```python
from build123d import *

# Parameters (mm, degrees)
SKETCH_4_R             = 12.471621376
EXTRUDE_2_DEPTH        = 8
SKETCH_6_R             = 8.974783973
EXTRUDE_3_DEPTH        = 8
HOLE_WIZARD_M201_D     = 20.25
HOLE_WIZARD_M201_DEPTH = 10
HOLE_WIZARD_M201_TIP   = 6.083713768


with BuildPart() as part:
    # Эскиз2 → Повернуть1 (revolve)
    with BuildSketch(Plane.XY):
        with BuildLine():
            Line((-4.5, 0.130191103), (-7.868865891, 0.130191103))
            ThreePointArc((-7.868865891, 0.130191103), (-9.846990335, 0.874747979), (-10.843230675, 2.73884198))
            Line((-10.843230675, 2.73884198), (-12.471621376, 15.115075065))
            Line((-12.471621376, 15.115075065), (-12.471621376, 23.115075065))
            Line((-12.471621376, 23.115075065), (-14.984883962, 23.115075065))
            Line((-14.984883962, 23.115075065), (-14.984883962, 29.115075065))
            Line((-14.984883962, 29.115075065), (-13.983803036, 29.115075065))
            Line((-13.983803036, 29.115075065), (-13.983803036, 32.115075065))
            Line((-13.983803036, 32.115075065), (-11.48027645, 32.115075065))
            Line((-11.48027645, 32.115075065), (-11.48027645, 37.115075065))
            Line((-11.48027645, 37.115075065), (-8.974783973, 37.115075065))
            Line((-8.974783973, 37.115075065), (-8.974783973, 23.115075065))
            Line((-8.974783973, 23.115075065), (-6.974783973, 23.115075065))
            Line((-6.974783973, 23.115075065), (-6.974783973, 18.115075065))
            Line((-6.974783973, 18.115075065), (-4.449353589, 18.115075065))
            Line((-4.449353589, 18.115075065), (-4.490567157, 3.479857527))
            Line((-4.490567157, 3.479857527), (-6.488062408, 3.489211927))
            Line((-6.488062408, 3.489211927), (-6.49087648, 2.489915788))
            Line((-6.49087648, 2.489915788), (-4.493381229, 2.480561388))
            Line((-4.493381229, 2.480561388), (-4.5, 0.130191103))
        make_face()
    revolve(axis=Axis((0, 0, 0), (0, 1, 0)))

    # Эскиз4 → Бобышка-Вытянуть2 (add)
    with BuildSketch(Plane(origin=(0, 23.115075065, 0), x_dir=(-1, 0, 0), z_dir=(0, -1, 0))):
        Polygon((-13.044923547, -7.374057026), (-0.13634106, -14.984263695), (12.908582486, -7.610206669), (13.044923547, 7.374057026), (0.13634106, 14.984263695), (-12.908582486, 7.610206669), align=None)
        Circle(SKETCH_4_R, mode=Mode.SUBTRACT)
    extrude(amount=EXTRUDE_2_DEPTH)

    # Эскиз6 → Бобышка-Вытянуть3 (add)
    with BuildSketch(Plane(origin=(0, 37.115075065, 0), x_dir=(1, 0, 0), z_dir=(0, 1, 0))):
        Circle(SKETCH_6_R)
    extrude(amount=-EXTRUDE_3_DEPTH)

    # Сверло под метчик  спиральное M201
    with Locations(Plane(origin=(0, 37.115075065, 0), x_dir=(1, 0, 0), z_dir=(0, 1, 0))):
        with Locations((0, 0)):
            Hole(HOLE_WIZARD_M201_D / 2, depth=HOLE_WIZARD_M201_DEPTH)
            with Locations((0, 0, -(HOLE_WIZARD_M201_DEPTH + HOLE_WIZARD_M201_TIP / 2))):  # 118° drill point
                Cone(0, HOLE_WIZARD_M201_D / 2, HOLE_WIZARD_M201_TIP, mode=Mode.SUBTRACT)


solid = part.part
```
Input: part model. Units: mm. Frame: model coordinates. A direction names the side the tool comes from. Give positions to 0.01 mm unless a question says otherwise; leave off trailing zeros. Write each loop counter-clockwise with the first axis right and the second up, starting at its lowest first coordinate (ties: lowest second). Pieces come first, ordered by that corner, then holes. Notation, with made-up numbers: (-28, 40) - (12, 40) arc R26 cw to (12, 59) - close; hole circle Ø1 at (36.25, -39.75). An arc over 180 degrees is marked (long way). Write item = value, one per line. Start each with the question number.
1) Cut plane A-A (y = 33.5). Return loops of the section in (x, z) (3 decimals).
2) Reachability of faces 1 (the face through (-7, 23.115, 12)), 2 (the face through (-10, 29.115, -10)), 3 (the face through (-7, 23.115, -12)), 4 (the face through (6.29, 19.17, -11.35)), 5 (the face through (7, 23.115, 12)) from +Z, -Z, +X, -X, +Y, -Y: full face, straight path, thin tool, end or side. Return the list, or none.
3) Material intervals for L1, parallel to Z at x = 0, y = 24.9; L2, parallel to Y at x = 7, z = -10.5; L3, parallel to Y at x = -3.5, z = -4.25, sorted ascending. Write a range as [from, to].
4) Pin query (flat end, axial travel): pin 1 (2.5 mm diameter, centred on x = 4.5, z = 9.5, fed in from -Y); pin 2 (10 mm diameter, centred on y = 10.5, z = -7.5, fed in from +X); pin 3 (5 mm diameter, centred on y = 5, z = 8.5, fed in from -X); pin 4 (8.5 mm diameter, centred on x = 0, z = 0, fed in from -Y). Return the tip coordinate at first contact, or that it passes through.
5) Draft query along X for faces 6 (the face through (-6.29, 19.17, 11.35)), 7 (the face through (0, 18.115, -5)), 8 (the face through (6.681, 19.171, 11.126)), 9 (the face through (-4.264, 10.695, 1.343)). Return one class per face: pulls with the +X half, pulls with the -X half, needs draft (parallel to the pull), parting line crosses it, or undercut.
6) Cut plane B-B (y = 6.5). Return loops of the section in (x, z).
Answers follow:
q1.outline = circle Ø22.961 at (0, 0); hole circle Ø20.25 at (0, 0)
q2.face_1 = +Z, -X, -Y
q2.face_2 = +Y
q2.face_3 = -Z, -X, -Y
q2.face_4 = -Z, +X, -Y
q2.face_5 = +Z, +X, -Y
q3.L1 = [-14.98, -8.97], [8.97, 14.98]
q3.L2 = [15.12, 32.12]
q3.L3 = [0.13, 2.49], [3.48, 18.12]
q4.pin_1 = 0.47
q4.pin_2 = 12.93
q4.pin_3 = -9.43
q4.pin_4 = through
q5.face_6 = pulls with the -X half
q5.face_7 = undercut
q5.face_8 = pulls with the +X half
q5.face_9 = undercut
q6.outline = circle Ø22.68 at (0, 0); hole circle Ø8.96 at (0, 0)
